Part model, mm, in its own coordinate system. A direction names the side the tool comes from. Give positions to 0.01 mm unless a question says otherwise; leave off trailing zeros. Write each loop counter-clockwise with the first axis right and the second up, starting at its lowest first coordinate (ties: lowest second). Pieces come first, ordered by that corner, then holes. Notation, with made-up numbers: M 65,-8.75 L 108,-8.75 A24 ccw 108,17.25 Z; hole C 42,83 d1. An arc over 180 degrees is marked long. Answer as CSV lines item,"result". Start each with the question number.
Item 1: Band-saw the part on B-B, the plane y = 18.5. List the corners of the cut face in (x, z), then the cut area to 3 significant figures.
Item 2: 3-axis set-ups, long thin cutter, end or side, ignore diameter. For faces 1 (the flat face through (101, 2, 3)), 2 (the flat face through (100, 2.465, 5)), 3 (the flat face through (118.3, 6.74, 1.98)), 4 (the flat face through (164, 8, 1.8)): which of +Z, -Z, +X, -X, +Y, -Y reach the whole face in a straight line?
Item 3: Band-saw the part on C-C, the plane x = 157.5. List the corners of the cut face in (y, z).
Item 4: Pin check, flat tips, straight feed: pin 1 (1 mm diameter, centred on y = 5.5, z = 2.5, fed in from -X); pin 2 (3 mm diameter, centred on x = 79.5, z = 1.5, fed in from -Y); pin 3 (3 mm diameter, centred on x = 162.5, y = 7.5, fed in from -Z); pin 4 (6 mm diameter, centred on y = 10, z = 6, fed in from -X). Stop position of each tip, or through.
Item 5: Wall check: L1, parallel to Z at x = 29.5, y = 18.25; L2, parallel to Y at x = 101, z = 5.75 (3 decimals); L3, parallel to X at y = 10.5, z = 1.5. Give the ranges that are in metal, low to high. Write a range as from..to.
Item 6: Band-saw the part on A-A, the plane x = 123.5. List the corners of the cut face in (y, z) (3 decimals).
Item 7: Two-plate mould, pull along X, no slides. Class faces 5 (the flat face through (198.054, 5.348, 2.754)), 6 (the flat face through (36, 8, 1.8)), 7 (the flat face through (99, 16, 0)): +X half, -X half, draft (parallel to the pull), parting line (faces both ways), or undercut.
from build123d import *

# Parameters (mm, degrees)
BOSS_EXTRUDE1_DEPTH = 200
CUT_EXTRUDE1_DEPTH  = 202.45470955
CUT_EXTRUDE2_DEPTH  = 202.45470955
BOSS_EXTRUDE2_REACH = 203.455
SKETCH5_W           = 3
SKETCH5_H           = 5
CUT_EXTRUDE3_DEPTH  = 202.45470955
CUT_EXTRUDE4_DEPTH  = 1.8
SKETCH9_W           = 19.4
SKETCH9_H           = 11.2
SKETCH9_W_2         = 15.4
SKETCH9_H_2         = 7.2
CUT_EXTRUDE6_DEPTH  = 202.45470955
CUT_EXTRUDE8_START  = -6.8
SKETCH10_W          = 19.4
SKETCH10_H          = 11.2
SKETCH10_W_2        = 15.4
SKETCH10_H_2        = 7.2
CUT_EXTRUDE8_DEPTH  = 22.6
SKETCH11_W          = 19.4
SKETCH11_H          = 12.8
SKETCH11_W_2        = 15.4
SKETCH11_H_2        = 8.8
CUT_EXTRUDE9_DEPTH  = 97.8


with BuildPart() as part:
    # Sketch1 → Boss-Extrude1 (new body)
    with BuildSketch(Plane(origin=(0, 0, 0), x_dir=(0, 0, -1), z_dir=(1, 0, 0))):
        Polygon((0, 0), (-10, 0), (0, 22), align=None)
    extrude(amount=BOSS_EXTRUDE1_DEPTH)

    # Sketch2 → Cut-Extrude1 (cut, through all)
    with BuildSketch(Plane(origin=(200, 0, 0), x_dir=(0, 0, -1), z_dir=(1, 0, 0))):
        with BuildLine():
            Line((-10, 0), (-0.5, 20.9))
            ThreePointArc((-0.5, 20.9), (-2.709071222, 9.295032374), (-10, 0))
        make_face()
    extrude(amount=-CUT_EXTRUDE1_DEPTH, mode=Mode.SUBTRACT)

    # Sketch4 → Cut-Extrude2 (cut, through all)
    with BuildSketch(Plane(origin=(200, 0, 0), x_dir=(0, 0, -1), z_dir=(1, 0, 0))):
        Polygon((-5, 0), (0, 5), (0, 0), align=None)
    extrude(amount=-CUT_EXTRUDE2_DEPTH, mode=Mode.SUBTRACT)

    # Boss-Extrude2: up to this face of the body (flat: up to its plane)
    boss_extrude2_end = Plane(part.part.faces().sort_by_distance((100, 2.5, 2.5))[0])
    # Sketch5 → Boss-Extrude2 (add, up to the picked face)
    with BuildSketch(Plane(origin=(0, 0, 0), x_dir=(-1, 0, 0), z_dir=(0, 0, -1)), mode=Mode.PRIVATE) as boss_extrude2_sk1:
        with Locations((-198.5, 2.5)):
            Rectangle(SKETCH5_W, SKETCH5_H)
    boss_extrude2_tool1 = split(extrude(boss_extrude2_sk1.sketch, amount=-BOSS_EXTRUDE2_REACH, mode=Mode.PRIVATE), bisect_by=boss_extrude2_end, keep=Keep.BOTH, mode=Mode.PRIVATE)
    boss_extrude2 = boss_extrude2_tool1.solids().sort_by(Axis((198.5, 2.5, 0), (0, 0, 1)))[0]
    add(boss_extrude2)

    # Sketch6 → Cut-Extrude3 (cut, through all)
    with BuildSketch(Plane(origin=(0, 0, 0), x_dir=(-1, 0, 0), z_dir=(0, 0, -1))):
        Polygon((-200, 22), (-191.992654846, 22), (-200, 0), align=None)
    cut_extrude3 = extrude(amount=-CUT_EXTRUDE3_DEPTH, mode=Mode.SUBTRACT)

    # Mirror2: Boss-Extrude2, Cut-Extrude3 across plane
    add(boss_extrude2.mirror(Plane(origin=(100, 0, 0), x_dir=(0, 0, 1), z_dir=(1, 0, 0))))
    add(cut_extrude3.mirror(Plane(origin=(100, 0, 0), x_dir=(0, 0, 1), z_dir=(1, 0, 0))), mode=Mode.SUBTRACT)

    # Sketch8 → Cut-Extrude4 (cut)
    with BuildSketch(Plane(origin=(0, 0, 0), x_dir=(-1, 0, 0), z_dir=(0, 0, -1))):
        Polygon((-165.621385956, 11.1), (-167.411171791, 8), (-165.621385956, 4.9), (-162.041814288, 4.9), (-160.252028453, 8), (-162.041814288, 11.1), align=None)
    cut_extrude4 = extrude(amount=-CUT_EXTRUDE4_DEPTH, mode=Mode.SUBTRACT)

    # Sketch9 → Cut-Extrude6 (cut, through all)
    with BuildSketch(Plane.XY):
        with Locations((99.915800061, 8.065)):
            Rectangle(SKETCH9_W, SKETCH9_H)
        with Locations((99.915800061, 8.065)):
            Rectangle(SKETCH9_W_2, SKETCH9_H_2, mode=Mode.SUBTRACT)
    extrude(amount=CUT_EXTRUDE6_DEPTH, mode=Mode.SUBTRACT)


with BuildPart() as cut_extrude6_kept_piece:
    # of the separate pieces the step leaves, the one the design keeps (cut_extrude6_pieces_kept)
    add(part.part.solids().sort_by_distance((197, 5, 0))[0])

    # Sketch10 → Cut-Extrude8 (cut)
    # profile 1 of 2: a face of its own
    with BuildSketch(Plane(origin=(32.136000823, 0, -55.661186177), x_dir=(0.866025403784433, 0, 0.5000000000000099), z_dir=(-0.5000000000000098, 0, 0.8660254037844329)).offset(CUT_EXTRUDE8_START)):
        with Locations((113.139032853, 8.065)):
            Rectangle(SKETCH10_W, SKETCH10_H)
        with Locations((113.139032853, 8.065)):
            Rectangle(SKETCH10_W_2, SKETCH10_H_2, mode=Mode.SUBTRACT)
    # profile 2 of 2: a face of its own
    with BuildSketch(Plane(origin=(32.136000823, 0, -55.661186177), x_dir=(0.866025403784433, 0, 0.5000000000000099), z_dir=(-0.5000000000000098, 0, 0.8660254037844329)).offset(CUT_EXTRUDE8_START)):
        with Locations((113.139032853, 8.065)):
            Rectangle(SKETCH10_W_2, SKETCH10_H_2)
    cut_extrude8 = extrude(amount=CUT_EXTRUDE8_DEPTH, mode=Mode.SUBTRACT)

    # Sketch11 → Cut-Extrude9 (cut)
    # profile 1 of 2: a face of its own
    with BuildSketch(Plane(origin=(115.669713788, 0, -66.781940393), x_dir=(0.4999999999999981, -1.9080601945838373e-15, 0.8660254037844397), z_dir=(-0.8660254037844397, 3.3048572009189827e-15, 0.4999999999999981))):
        with Locations((60.371690641, 23.065)):
            Rectangle(SKETCH11_W, SKETCH11_H)
        with Locations((60.371690641, 23.065)):
            Rectangle(SKETCH11_W_2, SKETCH11_H_2, mode=Mode.SUBTRACT)
    # profile 2 of 2: a face of its own
    with BuildSketch(Plane(origin=(115.669713788, 0, -66.781940393), x_dir=(0.4999999999999981, -1.9080601945838373e-15, 0.8660254037844397), z_dir=(-0.8660254037844397, 3.3048572009189827e-15, 0.4999999999999981))):
        with Locations((60.371690641, 23.065)):
            Rectangle(SKETCH11_W_2, SKETCH11_H_2)
    cut_extrude9 = extrude(amount=CUT_EXTRUDE9_DEPTH, mode=Mode.SUBTRACT)

    # Mirror4: Cut-Extrude8, Cut-Extrude9 across plane
    add(cut_extrude8.mirror(Plane(origin=(100, 0, 0), x_dir=(0, 0, 1), z_dir=(1, 0, 0))), mode=Mode.SUBTRACT)
    add(cut_extrude9.mirror(Plane(origin=(100, 0, 0), x_dir=(0, 0, 1), z_dir=(1, 0, 0))), mode=Mode.SUBTRACT)

    # Mirror5: Cut-Extrude4 across plane
    add(cut_extrude4.mirror(Plane(origin=(100, 0, 0), x_dir=(0, 0, 1), z_dir=(1, 0, 0))), mode=Mode.SUBTRACT)


solid = cut_extrude6_kept_piece.part
Output:
1,outline,"M 6.73,0 L 59.86,0 L 60.71,0.49 L 6.73,0.49 Z; M 98.66,0 L 101.34,0 L 100.49,0.49 L 99.51,0.49 Z; M 139.29,0.49 L 140.14,0 L 193.27,0 L 193.27,0.49 Z"
1,area,"53.8 mm²"
2,face 1,"-Z, -Y"
2,face 2,"+Z, -Z, +Y"
2,face 3,"+Z"
2,face 4,"-Z"
3,outline,"M 0,5 L 5,0 L 22,0 L 20.9,0.5 A25 cw 0,10 Z"
4,pin 1,"x = 1.82"
4,pin 2,"y = 2"
4,pin 3,"z = 1.8"
4,pin 4,"through"
5,L1,"0..0.51"
5,L2,"0..2.465"
5,L3,"3.82..34.03, 38.3..59.02, 81.42..90.22, 109.62..118.58, 140.98..161.7, 165.97..196.18"
6,outline,"M 0,5 L 2.465,2.535 L 2.465,7.302 A25 cw 0,10 Z; M 13.665,0 L 16.665,0 L 16.665,0.646 A25 cw 13.665,1.193 Z"
7,face 5,"+X half"
7,face 6,"undercut"
7,face 7,"draft"
